```python
from build123d import *

# Parameters (mm, degrees)
SKETCH1_R               = 4
EXTRUDE1_DEPTH          = 100
CHAMFER1_SIZE           = 0.8
SKETCH2_W               = 103.982490854
SKETCH2_H               = 8.719679173
CUT_EXTRUDE1_DEPTH      = 5
CUT_EXTRUDE1_DEPTH_BACK = 5
CHAMFER2_SIZE           = 0.8


with BuildPart() as part:
    # Sketch1 → Extrude1 (new body, symmetric)
    with BuildSketch(Plane.XY):
        Circle(SKETCH1_R)
    extrude(amount=EXTRUDE1_DEPTH, both=True)

    # Chamfer1
    chamfer1_edges = [part.edges().sort_by_distance(p)[0] for p in [
        (-4, 0, -100),
        (-4, 0, 100),
    ]]
    chamfer(chamfer1_edges, length=CHAMFER1_SIZE)

    # Sketch2 → Cut-Extrude1 (cut, two sides)
    with BuildSketch(Plane(origin=(0, 0, 0), x_dir=(0, 0, -1), z_dir=(1, 0, 0))) as cut_extrude1_sk:
        with Locations((51.991245427, -0.359839587)):
            Rectangle(SKETCH2_W, SKETCH2_H)
    extrude(amount=CUT_EXTRUDE1_DEPTH, mode=Mode.SUBTRACT)
    extrude(cut_extrude1_sk.sketch, amount=-CUT_EXTRUDE1_DEPTH_BACK, mode=Mode.SUBTRACT)

    # Chamfer2
    chamfer2_edges = [part.edges().sort_by_distance(p)[0] for p in [
        (-4, 0, 0),
    ]]
    chamfer(chamfer2_edges, length=CHAMFER2_SIZE)


solid = part.part
```
For this review, take the finished solid that the model builds, in its own axes (mm). Give positions to 0.01 mm unless a question says otherwise; leave off trailing zeros. Write each loop counter-clockwise with the first axis right and the second up, starting at its lowest first coordinate (ties: lowest second). Pieces come first, ordered by that corner, then holes. Notation, with made-up numbers: M 77.5,-0.75 L 89.5,-0.75 A18 cw 89.5,6.25 Z; hole C 44.25,17 d5. An arc over 180 degrees is marked long. Answer as a JSON object with one key per item and string values. Group by question number.
Item 1: For pin 1 Ø1.5 at (x, z) = (-3, 15.5) entering from +Y; pin 2 Ø1.5 at (y, z) = (-2, 72) entering from +X, all flat-tipped, find the tip position at first contact; note any pin that passes through.
Item 2: Consider section A-A on z = 58.5. Write out the cut boundary in (x, y).
Item 3: For probe 1 along X at (y, z) = (3.5, 39.5); probe 2 along Y at (x, z) = (-1.25, 11.5); probe 3 along X at (y, z) = (-1.5, 83.5), list the stretches that pass through material, from the lowest coordinate up. Write a range as [from, to].
Check result:
{
 "1": {"pin 1": "stops at y = 3.31", "pin 2": "stops at x = 3.8"},
 "2": {"outline": "C 0,0 d8"},
 "3": {"probe 1": "x = [-1.94, 1.94]", "probe 2": "y = [-3.8, 3.8]", "probe 3": "x = [-3.71, 3.71]"}
}
